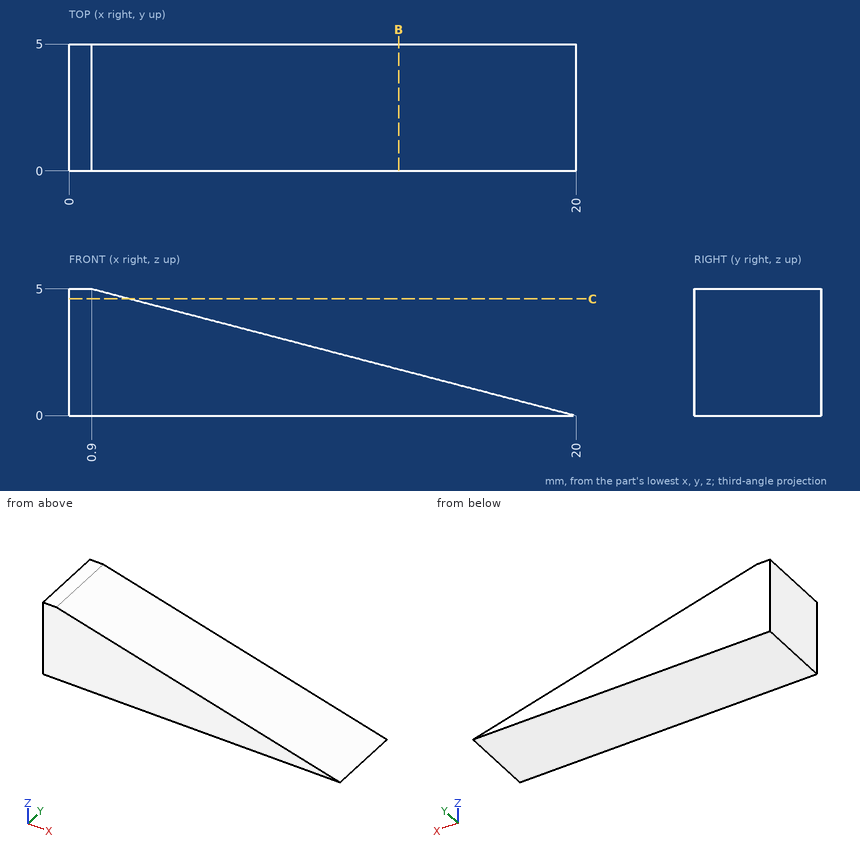
Input: dimensioned drawing with shaded views. Units: mm. Origin: part minimum x, y, z. Coordinates: 2 decimals unless noted, no trailing zeros. Order: outer loops, then holes, each group sorted by start corner. A loop starts at its lowest first (then second) coordinate and runs counter-clockwise, first axis right, second up. Notation, with made-up numbers: (9.5, 81.25) - (37.5, 81.25) arc R19 cw to (37.5, 89.25) - close; hole circle Ø1 at (33.5, -23.5). An arc over 180 degrees is marked (long way). Put each result on its own line as item: value.
1. Cut plane B-B on x = 13. Return the cut outline in (y, z).
Report:
outline: (0, 0) - (5, 0) - (5, 1.83) - (0, 1.83) - close
2. Cut plane C-C on z = 4.6. Return the cut outline in (x, y), then the cut area to 3 significant figures.
Report:
outline: (0, 0) - (2.43, 0) - (2.43, 5) - (0, 5) - close
area: 12.1 mm2
3. Contact query for flat-ended pins moving along their axis: pin 1 Ø2 at (y, z) = (2.5, 1.5) entering from -X; pin 2 Ø1.5 at (x, y) = (15.5, 2) entering from +Z; pin 3 Ø1 at (x, z) = (11, 4) entering from +Y. Output: stop coordinate, or through.
Report:
pin 1: stops at x = 0
pin 2: stops at z = 1.37
pin 3: passes through
4. Line query: line 1 along Z through (x, y) = (8.5, 4.35); line 2 along Z through (x, y) = (6.5, 3). Output: solid intervals per line, ascending.
Report:
line 1: z = 0 to 3.01
line 2: z = 0 to 3.53
